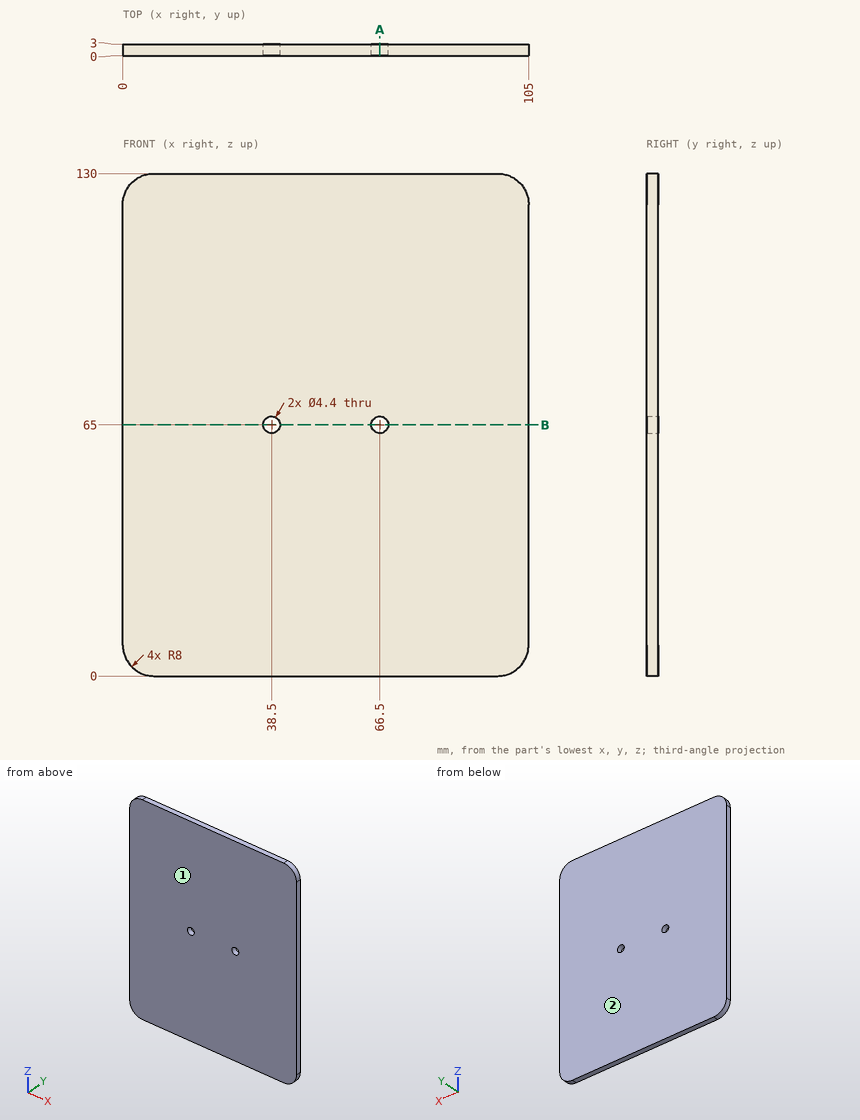
Here's the drawing with two shaded views (mm, measured from the low corner). I have some questions. Round coordinates to 2 decimals unless told otherwise and drop trailing zeros. Loops run counter-clockwise (first coordinate to the right, second up) from the corner with the lowest first, then second, coordinate; pieces in that order, holes last.
Item 1: Please list where these lines run through material, in increasing order: L1, parallel to Z at x = 38.5, y = 2.05; L2, parallel to Z at x = 37, y = 0.5; L3, parallel to Z at x = 100.5, y = 1.95.
Item 2: Suppose I cut it at A-A, the plane x = 66.5. Write out the boundary of the cut face in (y, z), then the cut area to 3 significant figures.
Item 3: Suppose I cut it at B-B, the plane z = 65. Write out the boundary of the cut face in (x, y).
Item 4: If we mould it in two halves opening along Y, with no side actions, what happens to the marked faces 1 and 2? For each: +Y half, -Y half, draft (parallel to the pull), parting line (faces both ways), or undercut.
Reported:
1. L1: z = 0 to 62.8, 67.2 to 130
1. L2: z = 0 to 63.39, 66.61 to 130
1. L3: z = 0.81 to 129.19
2. outline: (0, 0) - (3, 0) - (3, 62.8) - (0, 62.8) - close; (0, 67.2) - (3, 67.2) - (3, 130) - (0, 130) - close
2. area: 377 mm2
3. outline: (0, 0) - (36.3, 0) - (36.3, 3) - (0, 3) - close; (40.7, 0) - (64.3, 0) - (64.3, 3) - (40.7, 3) - close; (68.7, 0) - (105, 0) - (105, 3) - (68.7, 3) - close
4. face 1: -Y half
4. face 2: +Y half
